CAD build for the part. Positions are in the model's coordinates, mm. Face numbers are marked on the shaded views. A direction names the side the tool comes from. Round coordinates to 2 decimals unless told otherwise and drop trailing zeros. Loops run counter-clockwise (first coordinate to the right, second up) from the corner with the lowest first, then second, coordinate; pieces in that order, holes last. Notation, with made-up numbers: (-19, -39.5) - (38, -39.5) arc R19 ccw to (38, -21.5) - close; hole circle Ø11 at (59, -36). An arc over 180 degrees is marked (long way). Use one line per item in the form item = value.
from build123d import *

# Parameters (mm, degrees)
SKETCH2_W           = 15.8
SKETCH2_H           = 15.8
BOSS_EXTRUDE2_DEPTH = 5.4
SKETCH4_W           = 13.4
SKETCH4_H           = 13.4
CUT_EXTRUDE1_DEPTH  = 3.2
SKETCH7_R           = 3.255
SKETCH7_R_2         = 2.4
BOSS_EXTRUDE5_DEPTH = 3.2
SKETCH8_R           = 5.15
CUT_EXTRUDE2_DEPTH  = 0.3
BOSS_EXTRUDE8_DEPTH = 2.8
CIRPATTERN1_COUNT   = 4
BOSS_EXTRUDE9_DEPTH = 2.9
REVOLVE4_ANGLE      = 50
CIRPATTERN9_COUNT   = 4


with BuildPart() as part:
    # Sketch2 → Boss-Extrude2 (new body)
    with BuildSketch(Plane(origin=(0, 0, 0), x_dir=(1, 0, 0), z_dir=(0, 1, 0))):
        with Locations((7.9, 7.9)):
            Rectangle(SKETCH2_W, SKETCH2_H)
    extrude(amount=-BOSS_EXTRUDE2_DEPTH)

    # Sketch4 → Cut-Extrude1 (cut)
    with BuildSketch(Plane(origin=(0, 0, 0), x_dir=(1, 0, 0), z_dir=(0, 1, 0))):
        with Locations((7.9, 7.9)):
            Rectangle(SKETCH4_W, SKETCH4_H)
    extrude(amount=-CUT_EXTRUDE1_DEPTH, mode=Mode.SUBTRACT)

    # Sketch7 → Boss-Extrude5 (add)
    with BuildSketch(Plane(origin=(0, -3.2, 0), x_dir=(1, 0, 0), z_dir=(0, 1, 0))):
        with Locations((7.85, 7.85)):
            Circle(SKETCH7_R)
        with Locations((7.85, 7.85)):
            Circle(SKETCH7_R_2, mode=Mode.SUBTRACT)
    extrude(amount=BOSS_EXTRUDE5_DEPTH)

    # Sketch8 → Cut-Extrude2 (cut)
    with BuildSketch(Plane(origin=(0, -5.4, 0), x_dir=(-1, 0, 0), z_dir=(0, -1, 0))):
        with Locations((-7.9, 7.9)):
            Circle(SKETCH8_R)
    extrude(amount=-CUT_EXTRUDE2_DEPTH, mode=Mode.SUBTRACT)

    # Sketch11 → Boss-Extrude8 (add)
    with BuildSketch(Plane.XZ.offset(5.4)):
        Polygon((11.683021279, -2.207790411), (12.637615434, -3.162384566), (13.203300859, -2.596699141), (12.248706704, -1.642104986), align=None)
        with BuildLine():
            ThreePointArc((11.585853022, -2.304958669), (12.133497372, -2.706975833), (12.637615434, -3.162384566))
            Line((12.637615434, -3.162384566), (11.683021279, -2.207790411))
            Line((11.683021279, -2.207790411), (11.585853022, -2.304958669))
        make_face()
        with BuildLine():
            ThreePointArc((10.459662524, -3.431149167), (11.028098464, -3.808851017), (11.541599923, -4.258400077))
            Line((11.541599923, -4.258400077), (12.637615434, -3.162384566))
            ThreePointArc((12.637615434, -3.162384566), (12.133497372, -2.706975833), (11.585853022, -2.304958669))
            Line((11.585853022, -2.304958669), (10.459662524, -3.431149167))
        make_face()
        with BuildLine():
            Line((12.637615434, -3.162384566), (11.541599923, -4.258400077))
            ThreePointArc((11.541599923, -4.258400077), (11.991148983, -4.771901536), (12.368850833, -5.340337476))
            Line((12.368850833, -5.340337476), (13.495041331, -4.214146978))
            ThreePointArc((13.495041331, -4.214146978), (13.093024167, -3.666502628), (12.637615434, -3.162384566))
        make_face()
        with BuildLine():
            Line((13.592209589, -4.116978721), (12.637615434, -3.162384566))
            ThreePointArc((12.637615434, -3.162384566), (13.093024167, -3.666502628), (13.495041331, -4.214146978))
            Line((13.495041331, -4.214146978), (13.592209589, -4.116978721))
        make_face()
        Polygon((13.203300859, -2.596699141), (12.637615434, -3.162384566), (13.592209589, -4.116978721), (14.157895014, -3.551293296), align=None)
    boss_extrude8 = extrude(amount=BOSS_EXTRUDE8_DEPTH)

    # CirPattern1: Boss-Extrude8 ×4 about axis
    cirpattern1_axis = Axis((7.9, 0, -7.9), (0, 1, 0))
    for i in range(1, CIRPATTERN1_COUNT):
        add(boss_extrude8.rotate(cirpattern1_axis, i * 360 / CIRPATTERN1_COUNT))

    # Sketch12 → Boss-Extrude9 (add)
    with BuildSketch(Plane.XZ.offset(5.4)):
        with BuildLine():
            Line((13.700369837, -5.195243125), (12.79406205, -5.617861387))
            ThreePointArc((12.79406205, -5.617861387), (13.3, -7.9), (12.79406205, -10.182138613))
            Line((12.79406205, -10.182138613), (13.700369837, -10.604756875))
            ThreePointArc((13.700369837, -10.604756875), (14.3, -7.9), (13.700369837, -5.195243125))
        make_face()
        with BuildLine():
            Line((10.604756875, -13.700369837), (10.182138613, -12.79406205))
            ThreePointArc((10.182138613, -12.79406205), (7.9, -13.3), (5.617861387, -12.79406205))
            Line((5.617861387, -12.79406205), (5.195243125, -13.700369837))
            ThreePointArc((5.195243125, -13.700369837), (7.9, -14.3), (10.604756875, -13.700369837))
        make_face()
        with BuildLine():
            Line((2.099630163, -10.604756875), (3.00593795, -10.182138613))
            ThreePointArc((3.00593795, -10.182138613), (2.5, -7.9), (3.00593795, -5.617861387))
            Line((3.00593795, -5.617861387), (2.099630163, -5.195243125))
            ThreePointArc((2.099630163, -5.195243125), (1.5, -7.9), (2.099630163, -10.604756875))
        make_face()
        with BuildLine():
            Line((5.195243125, -2.099630163), (5.617861387, -3.00593795))
            ThreePointArc((5.617861387, -3.00593795), (7.9, -2.5), (10.182138613, -3.00593795))
            Line((10.182138613, -3.00593795), (10.604756875, -2.099630163))
            ThreePointArc((10.604756875, -2.099630163), (7.9, -1.5), (5.195243125, -2.099630163))
        make_face()
    extrude(amount=BOSS_EXTRUDE9_DEPTH)

    # Sketch26 → Revolve4 (revolve)
    with BuildSketch(Plane(origin=(4.436864492, 0, -9.514886609), x_dir=(0.906307787, 0, 0.422618262), z_dir=(-0.422618262, 0, 0.906307787))):
        Polygon((10.22114725, -7.5), (10.82114725, -7.8), (10.22114725, -8.3), align=None)
    revolve4 = revolve(axis=Axis((7.9, -5.1, -7.9), (0, 1, 0)), revolution_arc=REVOLVE4_ANGLE)

    # CirPattern9: Revolve4 ×4 about axis
    cirpattern9_axis = Axis((7.9, -5.1, -7.9), (0, -1, 0))
    for i in range(1, CIRPATTERN9_COUNT):
        add(revolve4.rotate(cirpattern9_axis, i * 360 / CIRPATTERN9_COUNT))


solid = part.part
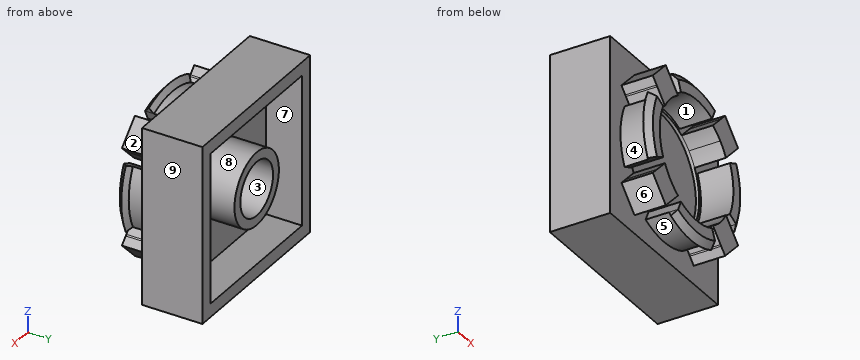
1) Tool access for the marked faces 1, 2, 3, 4 and 5: list every direction of +Z, -Z, +X, -X, +Y, -Y with a clear straight run to the whole face (end or side of a thin tool).
Report:
face_1 = -Y
face_2 = +Z, +X, -Y
face_3 = +Y
face_4 = -X
face_5 = -Z
2) Slice it at B-B (y = -6). State how many separate pieces and enclosed holes the cut face has, plus the area to 3 significant figures.
Report:
separate_pieces = 8
enclosed_holes = 0
area = 46.6 mm^2
3) Drill centre lines: probe 1 along X at (y, z) = (-0.95, -7.85) (3 decimals); probe 2 along Z at (x, y) = (7.85, -1.8) (3 decimals); probe 3 along X at (y, z) = (-5.3, -7.9). Where is each one in solid material? Low to high.
Report:
probe_1 = 0 to 1.2, 4.595 to 5.45, 10.25 to 11.105, 14.6 to 15.8
probe_2 = -15.8 to -14.6, -11.105 to -10.25, -5.45 to -4.595, -1.2 to 0
probe_3 = 0 to 2.75, 13.05 to 15.8
4) Slice it at A-A (y = -3). Write the cut outline in (x, z) (3 decimals).
Report:
outline = (0, -15.8) - (15.8, -15.8) - (15.8, 0) - (0, 0) - close; circle Ø6.51 at (7.85, -7.85); hole (1.2, -14.6) - (14.6, -14.6) - (14.6, -1.2) - (1.2, -1.2) - close; hole circle Ø4.8 at (7.85, -7.85)
5) Two-plate mould, pull along Z, no slides. Class the marked faces 6, 7, 8 and 9: +Z half, -Z half, draft (parallel to the pull), parting line (faces both ways), or undercut.
Report:
face_6 = -Z half
face_7 = undercut
face_8 = undercut
face_9 = draft
6) Flat gauge pins, fed straight in: pin 1 (1.8 mm diameter, centred on x = 11.5, z = -11.5, fed in from -Y); pin 2 (1.5 mm diameter, centred on x = 8, y = -7, fed in from +Z); pin 3 (8 mm diameter, centred on x = 7.5, z = -8.5, fed in from -Y). Where does each tip first touch, or does it go through?
Report:
pin_1 = -8.2
pin_2 = -1
pin_3 = -5.1
